```python
from build123d import *

# Parameters (mm, degrees)
BLOCK_SKETCH_W    = 20.6
BLOCK_SKETCH_H    = 20.6
BLOCK_DEPTH       = 10.3
ARM_X_SKETCH_W    = 25.8
ARM_X_SKETCH_H    = 11.124
ARM_Y_SKETCH_W    = 11.124
ARM_Y_SKETCH_H    = 25.8
SOCKET_X_SKETCH_W = 23.9
SOCKET_X_SKETCH_H = 6.35
SOCKET_Y_SKETCH_W = 6.35
SOCKET_Y_SKETCH_H = 23.9


with BuildPart() as part:
    # Block Sketch → Block (new, symmetric)
    with BuildSketch(Plane.XY):
        Rectangle(BLOCK_SKETCH_W, BLOCK_SKETCH_H)
    extrude(amount=BLOCK_DEPTH, both=True)

    # Arm X Sketch → Arm X (revolve)
    with BuildSketch(Plane.XY, mode=Mode.PRIVATE) as arm_x_sk:
        with Locations((23.2, 5.562)):
            Rectangle(ARM_X_SKETCH_W, ARM_X_SKETCH_H)
    revolve(arm_x_sk.sketch.rotate(Axis((-1000, 0, 0), (1, 0, 0)), 90), axis=Axis((-1000, 0, 0), (1, 0, 0)))

    # Arm Y Sketch → Arm Y (revolve)
    with BuildSketch(Plane.XY, mode=Mode.PRIVATE) as arm_y_sk:
        with Locations((5.562, 23.2)):
            Rectangle(ARM_Y_SKETCH_W, ARM_Y_SKETCH_H)
    revolve(arm_y_sk.sketch.rotate(Axis((0, -500, 0), (0, 1, 0)), 90), axis=Axis((0, -500, 0), (0, 1, 0)))

    # Socket X Sketch → Socket X (revolve, cut)
    with BuildSketch(Plane.XY, mode=Mode.PRIVATE) as socket_x_sk:
        with Locations((25.15, 3.175)):
            Rectangle(SOCKET_X_SKETCH_W, SOCKET_X_SKETCH_H)
    revolve(socket_x_sk.sketch.rotate(Axis((-1000, 0, 0), (1, 0, 0)), 90), axis=Axis((-1000, 0, 0), (1, 0, 0)), mode=Mode.SUBTRACT)

    # Socket Y Sketch → Socket Y (revolve, cut)
    with BuildSketch(Plane.XY, mode=Mode.PRIVATE) as socket_y_sk:
        with Locations((3.175, 25.15)):
            Rectangle(SOCKET_Y_SKETCH_W, SOCKET_Y_SKETCH_H)
    revolve(socket_y_sk.sketch.rotate(Axis((0, -500, 0), (0, 1, 0)), 90), axis=Axis((0, -500, 0), (0, 1, 0)), mode=Mode.SUBTRACT)


solid = part.part
```
Work out the finished part from the listing and answer in its coordinate system (mm). A direction names the side the tool comes from. Round coordinates to 2 decimals unless told otherwise and drop trailing zeros. Write each loop counter-clockwise with the first axis right and the second up, starting at its lowest first coordinate (ties: lowest second). Pieces come first, ordered by that corner, then holes. Notation, with made-up numbers: (78, 15) -> (109, 15) arc R31 ccw to (109, 50) -> close; hole circle Ø4 at (7.25, -14.5). An arc over 180 degrees is marked (long way). Write each question's results on one line, items separated by ' | '.
Q1. Section A-A, the plane y = 0 is taken. Write down the section's boundary in (x, z).
Data:
outline: (-10.3, -10.3) -> (10.3, -10.3) -> (10.3, -11.12) -> (36.1, -11.12) -> (36.1, -6.35) -> (13.2, -6.35) -> (13.2, 6.35) -> (36.1, 6.35) -> (36.1, 11.12) -> (10.3, 11.12) -> (10.3, 10.3) -> (-10.3, 10.3) -> close
Q2. Flat-ended cylindrical pins translate along their axes: P1, Ø2, axis at y = 26, z = -3.5, coming from the +X side; P2, Ø5, axis at y = 26.5, z = -4.5, coming from the +X side; P3, Ø4, axis at x = 2.5, z = -1.5, coming from the -Y side. Find the tip coordinate at first contact, or state that the pin passes through.
Data:
P1: x = 10.84 | P2: x = 10.94 | P3: y = -10.3
Q3. Straight lines are drawn through the part: line 1 along X through (y, z) = (25, 0); line 2 along X through (y, z) = (6, 1.75). For each, find the intervals that lie inside material, in ascending order. Write a range as [from, to].
Data:
line 1: [-11.12, -6.35], [6.35, 11.12] | line 2: [-10.3, 13.2]
Q4. Section D-D, the plane z = 0 is taken. Write down the section's boundary in (x, y), then the cut area to 3 significant figures.
Data:
outline: (-11.12, 10.3) -> (-10.3, 10.3) -> (-10.3, -10.3) -> (10.3, -10.3) -> (10.3, -11.12) -> (36.1, -11.12) -> (36.1, -6.35) -> (13.2, -6.35) -> (13.2, 6.35) -> (36.1, 6.35) -> (36.1, 11.12) -> (11.12, 11.12) -> (11.12, 36.1) -> (6.35, 36.1) -> (6.35, 13.2) -> (-6.35, 13.2) -> (-6.35, 36.1) -> (-11.12, 36.1) -> close | area: 990 mm^2
Q5. Section C-C, the plane y = 23.5 is taken. Write down the section's boundary in (x, z).
Data:
outline: circle Ø22.25 at (0, 0); hole circle Ø12.7 at (0, 0)
Q6. Determine the mould class of faces 1 (the cylindrical face through (3.86, 24.81, 5.04)), 2 (the flat face through (0, 0, -10.3)), 3 (the cylindrical face through (-3.34, 23.38, -10.61)), 4 (the flat face through (-10.3, 0, 0)) for opening direction Z: released by +Z, released by -Z, zero draft, split by the parting line, or undercut.
Data:
face 1: undercut | face 2: released by -Z | face 3: split by the parting line | face 4: zero draft
Q7. Which of the six approach directions +Z, -Z, +X, -X, +Y, -Y give full straight-line access (tool end or side, diameter ignored) to faces 5 (the flat face through (10.3, 9, -9)), 6 (the flat face through (9, 10.3, 9)), 7 (the flat face through (0, 0, 10.3)), 8 (the flat face through (-9, 10.3, 9)), 9 (the flat face through (13.2, 0, 0))?
Data:
face 5: -Z, +X, +Y | face 6: +Z, +X, +Y | face 7: +Z, -X, -Y | face 8: +Z, -X, +Y | face 9: +X
